Check sheet for the modelled part. Datum: model origin and axes. Units: mm. Face numbers are marked on the shaded views. Round coordinates to 2 decimals unless told otherwise and drop trailing zeros. Order: outer loops, then holes, each group sorted by start corner. A loop starts at its lowest first (then second) coordinate and runs counter-clockwise, first axis right, second up. Notation, with made-up numbers: (7, 79) -> (11, 79) arc R20 cw to (11, 115) -> close; hole circle Ø11 at (-14, 27). An arc over 180 degrees is marked (long way). Answer in a Markdown table with one row per item.
Autodesk Inventor part; units mm, degrees
ref_plane "YZ Plane" through (0, 0, 0) normal (1, 0, 0) x (0, 1, 0)
ref_plane "XZ Plane" through (0, 0, 0) normal (0, 1, 0) x (-1, 0, 0)
ref_plane "XY Plane" through (0, 0, 0) normal (0, 0, 1) x (1, 0, 0)
sketch "Sketch2" plane through (0, 0, 0) normal (0, 0, 1) x (1, 0, 0)
  line L0 (-10.4096, 0) -> (10.4096, 0) construction
  circle A0 centre (0, 0) radius 6.35
  circle A1 centre (21.7323, 0) radius 4.445
  circle A2 centre (-22.7937, 0) radius 4.445
  line L1 (-23.1652, 4.4294) -> (-0.5307, 6.3278)
  line L2 (22.1038, 4.4294) -> (-0.5307, 6.3278)
  line L3 (22.1038, -4.4294) -> (-0.5307, -6.3278)
  line L4 (-23.1652, -4.4294) -> (-0.5307, -6.3278)
  dimension "d4" = 12.7
  dimension "d5" = 8.89
  dimension "d6" = 8.89
extrude "Extrusion2" add sketch "Sketch2" along normal blind 2.159
sketch "Sketch3" plane through (0, 0, 2.159) normal (0, 0, 1) x (1, 0, 0)
  circle A0 centre (0, 0) radius 4.699
  dimension "d11" = 9.398
extrude "Extrusion3" add sketch "Sketch3" along normal blind 5.08
sketch "Sketch4" plane through (0, 0, 7.239) normal (0, 0, 1) x (1, 0, 0)
  circle A0 centre (0, 0) radius 2.54
  dimension "d14" = 5.08
extrude "Extrusion4" cut sketch "Sketch4" against normal through all
sketch "Sketch5" plane through (0, 0, 0) normal (0, 0, -1) x (-1, 0, 0)
  circle A0 centre (24.0637, 0) radius 0.635
  arc A1 (23.1652, -4.4294) -> (23.1652, 4.4294) centre (22.7937, 0) ccw
  line L0 (24.0637, 0) -> (4.699, 0)
  circle A2 centre (0, 0) radius 4.699
  circle A3 centre (20.8887, 0) radius 0.635
  circle A4 centre (17.7137, 0) radius 0.635
  circle A5 centre (14.5387, 0) radius 0.635
  circle A6 centre (11.3637, 0) radius 0.635
  line L1 (0, 0) -> (0, -5.8284)
  circle A7 centre (-24.0637, 0) radius 0.635
  circle A8 centre (-20.8887, 0) radius 0.635
  circle A9 centre (-17.7137, 0) radius 0.635
  circle A10 centre (-14.5387, 0) radius 0.635
  circle A11 centre (-11.3637, 0) radius 0.635
  dimension "d17" = 1.27
  dimension "d18" = 2.54
  dimension "d21" = 3.175
extrude "Extrusion5" cut sketch "Sketch5" against normal through all contours A0 | A6 L0 | L0 A6 | A5 L0 | L0 A5 | A4 L0 | L0 A4 | A3 L0 | L0 A3 | A7 | A8 | A9 | A10 | A11
equation "\"d6\" = d5"
properties part number "servo arm"
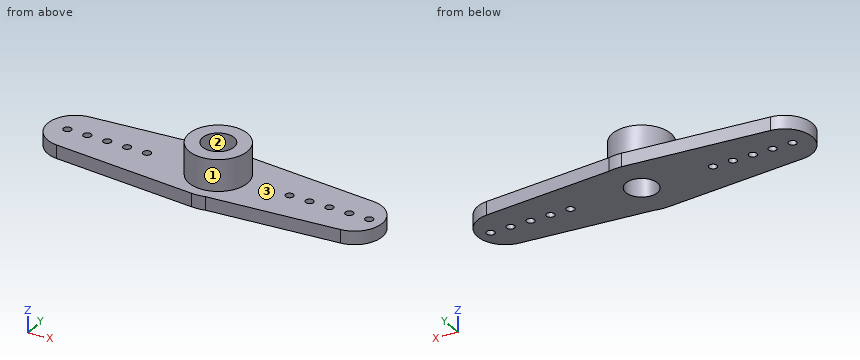
(1) Section check C-C on y = 0. Give the number of separate pieces and of enclosed holes in the cut face, plus the area to 3 significant figures.
Solutions:
| item | result |
|---|---|
| separate pieces | 12 |
| enclosed holes | 0 |
| area | 98.9 mm^2 |
(2) Scan lines: probe 1 along Z at (x, y) = (9, -4); probe 2 along Y at (x, z) = (-0.5, 4.75). Record each from-to range of solid material in increasing order. Write a range as from..to.
Solutions:
| item | result |
|---|---|
| probe 1 | 0..2.16 |
| probe 2 | -4.67..-2.49, 2.49..4.67 |
(3) Section check A-A on x = 0. Record the boundary of the cut face in (y, z), plus the area to 3 significant figures.
Solutions:
| item | result |
|---|---|
| outline | (-6.35, 0) -> (-2.54, 0) -> (-2.54, 7.24) -> (-4.7, 7.24) -> (-4.7, 2.16) -> (-6.35, 2.16) -> close; (2.54, 0) -> (6.35, 0) -> (6.35, 2.16) -> (4.7, 2.16) -> (4.7, 7.24) -> (2.54, 7.24) -> close |
| area | 38.4 mm^2 |
(4) Depth check by flat-ended pin: pin 1 Ø2 at (y, z) = (-1.5, 1) entering from -X; pin 2 Ø1.7 at (x, y) = (20.89, 0) entering from +Z; pin 3 Ø4 at (x, z) = (11.5, 2.5) entering from -Y. Enter the tip coordinate at first touch or a pass-through.
Solutions:
| item | result |
|---|---|
| pin 1 | x = -27.21 |
| pin 2 | z = 2.16 |
| pin 3 | y = -5.48 |
(5) Section check B-B on y = 2. Record the boundary of the cut face in (x, z), plus the area to 3 significant figures.
Solutions:
| item | result |
|---|---|
| outline | (-26.76, 0) -> (-1.57, 0) -> (-1.57, 7.24) -> (-4.25, 7.24) -> (-4.25, 2.16) -> (-26.76, 2.16) -> close; (1.57, 0) -> (25.7, 0) -> (25.7, 2.16) -> (4.25, 2.16) -> (4.25, 7.24) -> (1.57, 7.24) -> close |
| area | 134 mm^2 |
(6) Draft check along Y on the marked faces 1, 2 and 3. Enter one of: pulls with the +Y half, pulls with the -Y half, needs draft (parallel to the pull), parting line crosses it, or undercut.
Solutions:
| item | result |
|---|---|
| face 1 | parting line crosses it |
| face 2 | undercut |
| face 3 | needs draft |
(7) Section check D-D on z = 5.75. Record the boundary of the cut face in (x, y).
Solutions:
| item | result |
|---|---|
| outline | circle Ø9.4 at (0, 0); hole circle Ø5.08 at (0, 0) |
